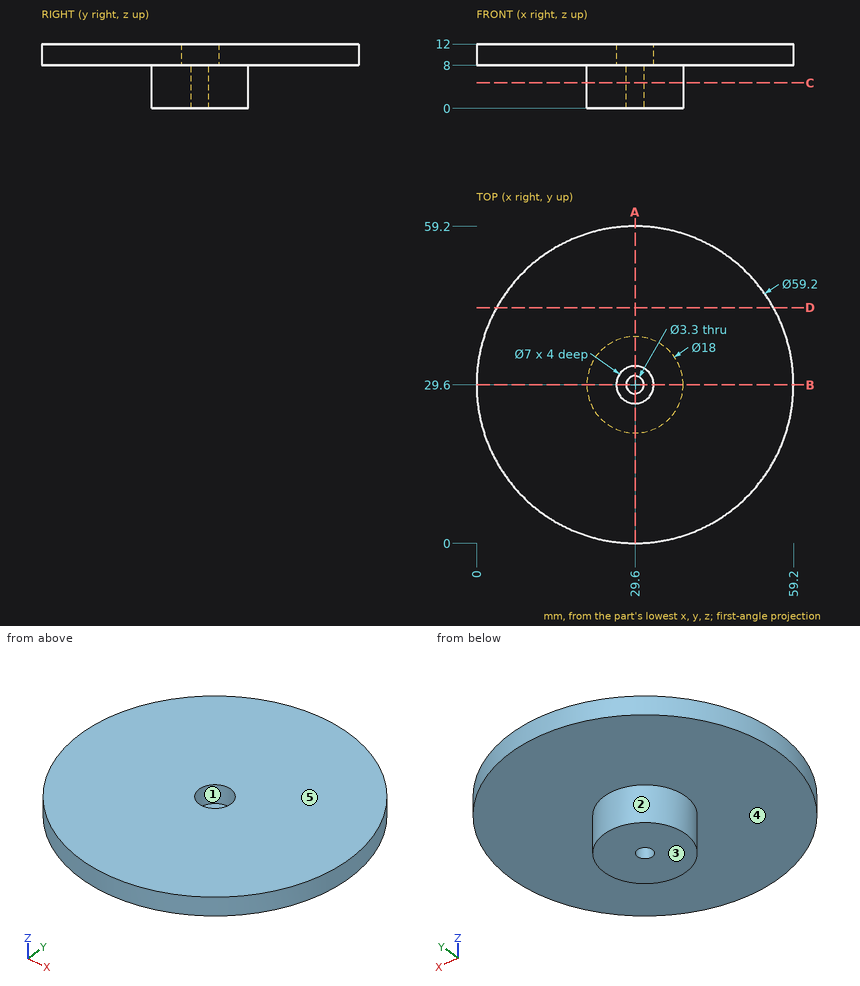
Drawing for the job (mm, zero at the part's lowest x, y, z). A direction names the side the tool comes from. Coordinates: 2 decimals unless noted, no trailing zeros. Write each loop counter-clockwise with the first axis right and the second up, starting at its lowest first coordinate (ties: lowest second). Pieces come first, ordered by that corner, then holes. Notation, with made-up numbers: (-10, 8.5) - (22, 8.5) arc R19 ccw to (22, 32.5) - close; hole circle Ø11 at (-26.75, -39.5). An arc over 180 degrees is marked (long way). Write each question's results on one line, items separated by ' | '. Start each with the question number.
1) 3-axis set-ups, long thin cutter, end or side, ignore diameter. For the marked faces 4 and 5: which of +Z, -Z, +X, -X, +Y, -Y reach the whole face in a straight line?
2) Mould opens along X. For the marked faces 1, 2 and 3 say: pulls with the +X half, pulls with the -X half, needs draft (parallel to the pull), parting line crosses it, or undercut.
3) Cut at A-A (x = 29.6). Write the cut outline in (y, z).
4) Flat gauge pins, fed straight in: P1, Ø1.5, axis at x = 30.5, z = 5.5, coming from the +Y side; P2, Ø1, axis at y = 16, z = 8.5, coming from the -X side; P3, Ø2, axis at y = 12.5, z = 8, coming from the +X side. Where does each tip first touch, or does it go through?
5) Cut at C-C (z = 4.75). Write the cut outline in (x, y), then the cut area to 3 significant figures.
6) Probe line 1 along Y through (x, z) = (29.6, 10.85); line 2 along Z through (x, y) = (24.5, 37.5). List the from-to ranges inside material, lowest first. Write a range as from..to.
7) Cut at D-D (y = 44). Write the cut outline in (x, z).
Returned:
1) face 4: -Z | face 5: +Z, +X, -X, +Y, -Y
2) face 1: undercut | face 2: parting line crosses it | face 3: needs draft
3) outline: (0, 8) - (20.6, 8) - (20.6, 0) - (27.95, 0) - (27.95, 8) - (26.1, 8) - (26.1, 12) - (0, 12) - close; (31.25, 0) - (38.6, 0) - (38.6, 8) - (59.2, 8) - (59.2, 12) - (33.1, 12) - (33.1, 8) - (31.25, 8) - close
4) P1: y = 38.6 | P2: x = 3.06 | P3: x = 54.44
5) outline: circle Ø18 at (29.6, 29.6); hole circle Ø3.3 at (29.6, 29.6) | area: 246 mm^2
6) line 1: 0..26.1, 33.1..59.2 | line 2: 8..12
7) outline: (3.74, 8) - (55.46, 8) - (55.46, 12) - (3.74, 12) - close
